```python
from build123d import *

# Parameters (mm, degrees)
BOSS_EXTRUDE1_DEPTH     = 40
BOSS_EXTRUDE2_START     = 30
SKETCH2_R               = 1.25
BOSS_EXTRUDE2_DEPTH     = 10
CUT_EXTRUDE1_DEPTH      = 91
CUT_EXTRUDE1_DEPTH_BACK = 91
SKETCH3_W               = 5
SKETCH3_H               = 5


with BuildPart() as part:
    # Sketch1 → Boss-Extrude1 (new, symmetric)
    with BuildSketch(Plane.XY):
        Polygon((0, 0), (80, 0), (80, 10), (75, 10), (75, 5), (0, 5), align=None)
    extrude(amount=BOSS_EXTRUDE1_DEPTH, both=True)

    # Sketch2 → Boss-Extrude2 (add)
    with BuildSketch(Plane.XY.offset(BOSS_EXTRUDE2_START)):
        with BuildLine():
            Line((0, 5), (-2.5, 5))
            ThreePointArc((-2.5, 5), (-5, 2.5), (-2.5, 0))
            Line((-2.5, 0), (0, 0))
            Line((0, 0), (0, 5))
        make_face()
        with Locations((-2.5, 2.5)):
            Circle(SKETCH2_R, mode=Mode.SUBTRACT)
    boss_extrude2 = extrude(amount=BOSS_EXTRUDE2_DEPTH)

    # Mirror2: Boss-Extrude2 across plane
    add(boss_extrude2.mirror(Plane.XY))

    # Sketch3 → Cut-Extrude1 (cut, two sides: drawn at the far end of the back side and taken through both)
    with BuildSketch(Plane.XY.offset(-CUT_EXTRUDE1_DEPTH_BACK)):
        with Locations((77.5, 7.5)):
            Rectangle(SKETCH3_W, SKETCH3_H)
    extrude(amount=CUT_EXTRUDE1_DEPTH + CUT_EXTRUDE1_DEPTH_BACK, mode=Mode.SUBTRACT)


solid = part.part
```
Geometry check sheet. Reference: the model listing, model coordinates, mm. A direction names the side the tool comes from. Give positions to 0.01 mm unless a question says otherwise; leave off trailing zeros. Write each loop counter-clockwise with the first axis right and the second up, starting at its lowest first coordinate (ties: lowest second). Pieces come first, ordered by that corner, then holes.
1) Access from +Z, -Z, +X, -X, +Y, -Y to the whole of each face (thin tool, end or side, straight path). Record for faces 1 (the cylindrical face through (-5, 2.6, -34.9)), 2 (the flat face through (-2, 4, 30)).
2) Release check for a two-part mould opening along Z. For faces 3 (the flat face through (80, 2, 1)), 4 (the flat face through (37, 3, 40)), 5 (the flat face through (-2, 4, -30)) record: pulls with the +Z half, pulls with the -Z half, needs draft (parallel to the pull), parting line crosses it, or undercut.
3) Section check A-A, the plane y = 2.5. Record the boundary of the cut face in (x, z), and give its area (3 significant figures).
4) Section check B-B, the plane z = 10. Record the boundary of the cut face in (x, y), and give its area (3 significant figures).
5) Gauge pin test, flat ends, axial feed: pin 1 (1.5 mm diameter, centred on x = -2.5, y = 2.5, fed in from +Z); pin 2 (1.5 mm diameter, centred on y = 3, z = 8, fed in from -X). Record the tip position at first contact, or that the pin passes through.
6) Material ranges on L1, parallel to Y at x = -2, z = 37; L2, parallel to X at y = 3.15, z = 9, recorded low to high.
Computed:
1. face 1: +Z, -Z, -X
1. face 2: -X, +Y, -Y
2. face 3: needs draft
2. face 4: pulls with the +Z half
2. face 5: undercut
3. outline: (-5, -40) - (-3.75, -40) - (-3.75, -30) - (-5, -30) - close; (-5, 30) - (-3.75, 30) - (-3.75, 40) - (-5, 40) - close; (-1.25, -40) - (80, -40) - (80, 40) - (-1.25, 40) - (-1.25, 30) - (0, 30) - (0, -30) - (-1.25, -30) - close
3. area: 6,450 mm2
4. outline: (0, 0) - (80, 0) - (80, 5) - (0, 5) - close
4. area: 400 mm2
5. pin 1: passes through
5. pin 2: stops at x = 0
6. L1: y = 0 to 1.35, 3.65 to 5
6. L2: x = 0 to 80
